from build123d import *

# Parameters (mm, degrees)
CROQUIS1_W                 = 31.5
CROQUIS1_H                 = 31.5
SALIENTE_EXTRUIR1_DEPTH    = 15
CROQUIS3_R                 = 10
CORTAR_EXTRUIR1_DEPTH      = 11.5
CROQUIS6_R                 = 1.75
CORTAR_EXTRUIR2_DEPTH      = 27.853770685
CORTAR_EXTRUIR3_REACH      = 40.279
CORTAR_EXTRUIR3_END_RADIUS = 10
CROQUIS7_R                 = 1
CORTAR_EXTRUIR4_REACH      = 40.279
CORTAR_EXTRUIR4_END_RADIUS = 10
CROQUIS8_R                 = 1
CROQUIS9_R                 = 1.4
CORTAR_EXTRUIR5_DEPTH      = 2.5
CROQUIS10_R                = 1.4
CORTAR_EXTRUIR6_DEPTH      = 2.5


with BuildPart() as part:
    # Croquis1 → Saliente-Extruir1 (new body)
    with BuildSketch(Plane(origin=(0, 0, 0), x_dir=(1, 0, 0), z_dir=(0, 1, 0))):
        Rectangle(CROQUIS1_W, CROQUIS1_H)
    extrude(amount=SALIENTE_EXTRUIR1_DEPTH)

    # Croquis3 → Cortar-Extruir1 (cut)
    with BuildSketch(Plane(origin=(0, 15, 0), x_dir=(1, 0, 0), z_dir=(0, 1, 0))):
        with Locations(Location((0, 0, 0), (0, 0, 270))):
            Circle(CROQUIS3_R)
    extrude(amount=-CORTAR_EXTRUIR1_DEPTH, mode=Mode.SUBTRACT)

    # Croquis6 → Cortar-Extruir2 (cut, through all)
    with BuildSketch(Plane(origin=(0, 15, 0), x_dir=(1, 0, 0), z_dir=(0, 1, 0))):
        with Locations(Location((-11.75, -11.75, 0), (0, 0, 270))):
            Circle(CROQUIS6_R)
        with Locations(Location((11.75, -11.75, 0), (0, 0, 90))):
            Circle(CROQUIS6_R)
        with Locations(Location((11.75, 11.75, 0), (0, 0, 270))):
            Circle(CROQUIS6_R)
        with Locations(Location((-11.75, 11.75, 0), (0, 0, 90))):
            Circle(CROQUIS6_R)
    extrude(amount=-CORTAR_EXTRUIR2_DEPTH, mode=Mode.SUBTRACT)

    # Cortar-Extruir3: up to this cylinder (the profile starts outside it)
    cortar_extruir3_end = Plane(origin=(0, 5, 0), z_dir=(0, 1, 0)) * Cylinder(CORTAR_EXTRUIR3_END_RADIUS, 101.558, mode=Mode.PRIVATE)
    # Croquis7 → Cortar-Extruir3 (cut, up to the surface)
    with BuildSketch(Plane.XY.offset(15.75), mode=Mode.PRIVATE) as cortar_extruir3_sk1:
        with Locations((0, 5)):
            Circle(CROQUIS7_R)
    cortar_extruir3_tool1 = extrude(cortar_extruir3_sk1.sketch, amount=-CORTAR_EXTRUIR3_REACH, mode=Mode.PRIVATE) - cortar_extruir3_end
    add(cortar_extruir3_tool1.solids().sort_by_distance((0, 5, 15.75))[0], mode=Mode.SUBTRACT)

    # Cortar-Extruir4: up to this cylinder (the profile starts outside it)
    cortar_extruir4_end = Plane(origin=(0, 13.123683, 0), z_dir=(0, 1, 0)) * Cylinder(CORTAR_EXTRUIR4_END_RADIUS, 101.558, mode=Mode.PRIVATE)
    # Croquis8 → Cortar-Extruir4 (cut, up to the surface)
    with BuildSketch(Plane(origin=(0, 0, -15.75), x_dir=(-1, 0, 0), z_dir=(0, 0, -1)), mode=Mode.PRIVATE) as cortar_extruir4_sk1:
        with Locations((0, 13.123683267)):
            Circle(CROQUIS8_R)
    cortar_extruir4_tool1 = extrude(cortar_extruir4_sk1.sketch, amount=-CORTAR_EXTRUIR4_REACH, mode=Mode.PRIVATE) - cortar_extruir4_end
    add(cortar_extruir4_tool1.solids().sort_by_distance((0, 13.123683, -15.75))[0], mode=Mode.SUBTRACT)

    # Croquis9 → Cortar-Extruir5 (cut)
    with BuildSketch(Plane.XY.offset(15.75)):
        with Locations((0, 5)):
            Circle(CROQUIS9_R)
    extrude(amount=-CORTAR_EXTRUIR5_DEPTH, mode=Mode.SUBTRACT)

    # Croquis10 → Cortar-Extruir6 (cut)
    with BuildSketch(Plane(origin=(0, 0, -15.75), x_dir=(-1, 0, 0), z_dir=(0, 0, -1))):
        with Locations((0, 13.123683267)):
            Circle(CROQUIS10_R)
    extrude(amount=-CORTAR_EXTRUIR6_DEPTH, mode=Mode.SUBTRACT)


solid = part.part
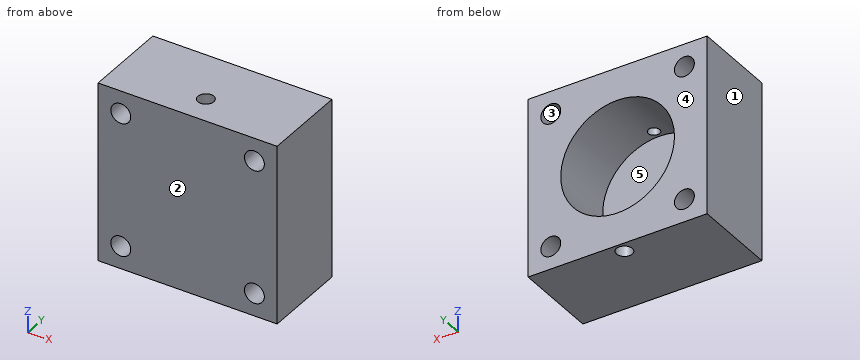
Here's how the part is built. I have some questions about the finished solid (model axes, mm). Face numbers are marked on the shaded views. A direction names the side the tool comes from. Round coordinates to 2 decimals unless told otherwise and drop trailing zeros. Order: outer loops, then holes, each group sorted by start corner. A loop starts at its lowest first (then second) coordinate and runs counter-clockwise, first axis right, second up. Notation, with made-up numbers: (57.25, -37.5) -> (73.25, -37.5) arc R17 ccw to (73.25, -4.5) -> close; hole circle Ø2 at (62, 48.5). An arc over 180 degrees is marked (long way). Return JSON: item names as keys, results as strings.
Q1. If we section it at C-C on y = 7: List the corners of the cut face in (x, z) for me, plus the area to 3 significant figures.
Filled sheet:
{"outline": "(-15.75, -15.75) -> (15.75, -15.75) -> (15.75, 15.75) -> (-15.75, 15.75) -> close; hole circle Ø3.5 at (-11.75, -11.75); hole circle Ø3.5 at (-11.75, 11.75); hole circle Ø20 at (0, 0); hole circle Ø3.5 at (11.75, -11.75); hole circle Ø3.5 at (11.75, 11.75)", "area": "640 mm^2"}
Q2. If we section it at D-D on y = 2.5: List the corners of the cut face in (x, z) for me, plus the area to 3 significant figures.
Filled sheet:
{"outline": "(-15.75, -15.75) -> (15.75, -15.75) -> (15.75, 15.75) -> (-15.75, 15.75) -> close; hole circle Ø3.5 at (-11.75, -11.75); hole circle Ø3.5 at (-11.75, 11.75); hole circle Ø3.5 at (11.75, -11.75); hole circle Ø3.5 at (11.75, 11.75)", "area": "954 mm^2"}
Q3. If we section it at A-A on z = -11.5: List the corners of the cut face in (x, y) for me.
Filled sheet:
{"outline": "(-15.75, 0) -> (-13.48, 0) -> (-13.48, 15) -> (-15.75, 15) -> close; (-10.02, 0) -> (10.02, 0) -> (10.02, 15) -> (-10.02, 15) -> close; (13.48, 0) -> (15.75, 0) -> (15.75, 15) -> (13.48, 15) -> close; hole circle Ø2 at (0, 13.12)"}
Q4. I need wall thicknesses on line 1 along Y through (x, z) = (0, 11.85); line 2 along X through (y, z) = (10.25, 11.75); line 3 along Y through (x, z) = (0, -10.65). Which ranges of each line are inside material? Lowest first, please. Write a range as from..to.
Filled sheet:
{"line 1": "y = 0..4, 6..15", "line 2": "x = -15.75..-13.5, -10..10, 13.5..15.75", "line 3": "y = 0..12.12, 14.12..15"}
Q5. If we section it at B-B on x = 0: List the corners of the cut face in (y, z) for me, plus the area to 4 significant figures.
Filled sheet:
{"outline": "(0, -15.75) -> (11.72, -15.75) -> (11.72, -13.25) -> (12.12, -13.25) -> (12.12, -10) -> (3.5, -10) -> (3.5, 10) -> (4, 10) -> (4, 13.25) -> (3.6, 13.25) -> (3.6, 15.75) -> (0, 15.75) -> close; (6, 10) -> (15, 10) -> (15, 15.75) -> (6.4, 15.75) -> (6.4, 13.25) -> (6, 13.25) -> close; (14.12, -13.25) -> (14.52, -13.25) -> (14.52, -15.75) -> (15, -15.75) -> (15, -10) -> (14.12, -10) -> close", "area": "215.5 mm^2"}
Q6. For pin 1 Ø1.5 at (x, z) = (0.5, -1) entering from -Y; pin 2 Ø12 at (x, z) = (0, 0) entering from +Y; pin 3 Ø2 at (x, z) = (11.75, -11.75) entering from +Y; pin 4 Ø1.2 at (x, y) = (0, 13.12) entering from -Z, each with a flat end and sliding along its axis, tell me the tip position at first contact or that it passes through.
Filled sheet:
{"pin 1": "stops at y = 0", "pin 2": "stops at y = 3.5", "pin 3": "passes through", "pin 4": "stops at z = 9.98"}
Q7. Which directions (+Z, -Z, +X, -X, +Y, -Y) give clear straight access to the entire face, cutting with the end or side of a thin tool? Please do the marked faces 4 and 5.
Filled sheet:
{"face 4": "+Z, -Z, +X, -X, +Y", "face 5": "+Y"}
Q8. If we mould it in two halves opening along X, with no side actions, what happens to the marked faces 1, 2 and 3? For each: released by +X, released by -X, zero draft, split by the parting line, or undercut.
Filled sheet:
{"face 1": "released by -X", "face 2": "zero draft", "face 3": "undercut"}
